Geometry check sheet. Reference: the model listing, model coordinates, mm. A direction names the side the tool comes from. Give positions to 0.01 mm unless a question says otherwise; leave off trailing zeros. Loops run counter-clockwise (first coordinate to the right, second up) from the corner with the lowest first, then second, coordinate; pieces in that order, holes last. Notation, with made-up numbers: (71, 30) -> (130, 30) arc R17 cw to (130, 55) -> close; hole circle Ø3 at (88, 9). An arc over 180 degrees is marked (long way). One line per question, with ' | ' between items.
from build123d import *

# Parameters (mm, degrees)
F0_W     = 50
F0_H     = 105
F1_DEPTH = 10
F2_R     = 1
F3_R     = 1
F4_T     = 1


# Not quite as in the source:
# - a shell that OpenCascade refuses in one call is made with other operations: the cavity is built on its own and cut out


with BuildPart() as f1:
    # F0 (on Front) → F1 (new body)
    with BuildSketch(Plane.XZ):
        with Locations((-25, 52.5)):
            Rectangle(F0_W, F0_H)
    extrude(amount=F1_DEPTH)

    # F2
    f2_edges = [f1.edges().sort_by_distance(p)[0] for p in [
        (-50, -5, 105),
        (0, -5, 105),
        (0, -5, 0),
        (-50, -5, 0),
    ]]
    fillet(f2_edges, radius=F2_R)

    # F3
    f3_edges = [f1.edges().sort_by_distance(p)[0] for p in [
        (-25, 0, 105),
    ]]
    fillet(f3_edges, radius=F3_R)

    # F4: shell of thickness 1, made by hand


with BuildPart() as f4_core1:
    # F4_t2: copy of F1
    add(f1.part)

    # the walls: a layer under each face that stays
    f4_faces = [f4_core1.faces().sort_by_distance(p)[0] for p in [
        (0, -5.5, 52.5),
        (-25, -5.5, 0),
        (-25, 0, 52.5),
        (-25, -5.5, 105),
        (-50, -5.5, 52.5),
    ]]
    thicken(f4_faces, amount=-F4_T, mode=Mode.SUBTRACT)


with BuildPart() as f1_1:
    add(f1.part)

    # what is left inside the walls is the cavity
    f4_cavity = [f4_core1.part.solids().sort_by_distance(p)[0] for p in [
        (-25, -1.01, 35.333333),
    ]]
    add(f4_cavity, mode=Mode.SUBTRACT)


solid = f1_1.part
Item 1: Release check for a two-part mould opening along Z. For faces 1 (the face through (-25, -5, 104)), 2 (the face through (-49.2, -10, 52.7)), 3 (the face through (-25, -5, 105)), 4 (the face through (-25, -5, 0)) record: pulls with the +Z half, pulls with the -Z half, needs draft (parallel to the pull), parting line crosses it, or undercut.
Result:
face 1: undercut | face 2: needs draft | face 3: pulls with the +Z half | face 4: pulls with the -Z half
Item 2: Sectioned sample at A-A (y = -7.5). Record the cut outline in (x, z), plus the area to 3 significant figures.
Result:
outline: (-50, 1) arc R1 ccw to (-49, 0) -> (-1, 0) arc R1 ccw to (0, 1) -> (0, 104) arc R1 ccw to (-1, 105) -> (-49, 105) arc R1 ccw to (-50, 104) -> close; hole (-49, 1) -> (-1, 1) -> (-1, 104) -> (-49, 104) -> close | area: 305 mm2
Item 3: Sectioned sample at C-C (x = -3). Record the cut outline in (y, z).
Result:
outline: (-10, 0) -> (-1, 0) arc R1 ccw to (0, 1) -> (0, 104) arc R1 ccw to (-1, 105) -> (-10, 105) -> (-10, 104) -> (-1, 104) -> (-1, 1) -> (-10, 1) -> close
Item 4: Sectioned sample at B-B (z = 34). Record the cut outline in (x, y).
Result:
outline: (-50, -10) -> (-49, -10) -> (-49, -1) -> (-1, -1) -> (-1, -10) -> (0, -10) -> (0, -1) arc R1 ccw to (-1, 0) -> (-49, 0) arc R1 ccw to (-50, -1) -> close
Item 5: Set-up check for faces 5 (the face through (-1, -5, 52)), 6 (the face through (-25, 0, 53)): record each of +Z, -Z, +X, -X, +Y, -Y from which the full face is reachable in a straight line by a thin tool's end or side.
Result:
face 5: -Y | face 6: +Z, -Z, +X, -X, +Y
Item 6: Scan lines: probe 1 along X at (y, z) = (-5.25, 40); probe 2 along Z at (x, y) = (-41.5, -5); probe 3 along Y at (x, z) = (-35.5, 37). Record each from-to range of solid material in increasing order.
Result:
probe 1: -50 to -49, -1 to 0 | probe 2: 0 to 1, 104 to 105 | probe 3: -1 to 0
Item 7: Depth check by flat-ended pin: pin 1 Ø5 at (x, z) = (-33, 68.5) entering from -Y. Enter the tip coordinate at first touch or a pass-through.
Result:
pin 1: y = -1
